The listing builds one solid part. Answer for the finished solid, in the listing's coordinates (mm). Give positions to 0.01 mm unless a question says otherwise; leave off trailing zeros. Order: outer loops, then holes, each group sorted by start corner. A loop starts at its lowest first (then second) coordinate and runs counter-clockwise, first axis right, second up. Notation, with made-up numbers: (13, 75) - (31, 75) arc R23 ccw to (31, 88) - close; hole circle Ø11 at (-11, 28). An arc over 180 degrees is marked (long way). Write each question's results on one line, items separated by ' | '. Start each with the question number.
1. Section A-A (x = 10) is taken. Give the vertices of the cut face in (y, z).
2. Find the intervals of material crossed by L1, parallel to Y at x = -63.55, z = 1.4; L2, parallel to Y at x = 40, z = 2.65; L3, parallel to Y at x = 87.1, z = 1.5, in increasing order.
3. Section B-B (z = 2.15) is taken. State how many separate pieces and enclosed holes the cut face has, and give its area (3 significant figures).
4. Determine the mould class of faces 1 (the face through (-66.498, -16.383, 1.972)), 2 (the face through (2, 27, 0)) for opening direction Y: released by +Y, released by -Y, zero draft, split by the parting line, or undercut.
5. Flat-ended cylindrical pins translate along their axes: pin 1 (4 mm diameter, centred on x = 63.55, y = 26.16, fed in from +Z); pin 2 (2 mm diameter, centred on x = 51, z = 2, fed in from -Y); pin 3 (4 mm diameter, centred on x = -40, y = -42.64, fed in from +Z); pin 4 (2 mm diameter, centred on y = -48.5, z = 1, fed in from +X). Find the tip coordinate at first contact, or state that the pin passes through.
from build123d import *

# Parameters (mm, degrees)
SKETCH1_R           = 1.5
SKETCH1_R_2         = 11
SKETCH1_R_3         = 4
SKETCH1_R_4         = 2.5
BOSS_EXTRUDE2_DEPTH = 4


with BuildPart() as part:
    # Sketch1 → Boss-Extrude2 (new body)
    with BuildSketch(Plane.XY):
        Polygon((-150.528484514, 102.663377685), (149.471515486, 102.663377685), (149.471515486, -47.336622315), (75.331349572, -47.336622315), (75.331349572, -51.336622315), (60.331349572, -51.336622315), (60.331349572, -47.336622315), (40.331349572, -47.336622315), (40.331349572, -51.336622315), (25.331349572, -51.336622315), (25.331349572, -47.336622315), (5.331349572, -47.336622315), (5.331349572, -51.336622315), (-9.668650428, -51.336622315), (-9.668650428, -47.336622315), (-29.668650428, -47.336622315), (-29.668650428, -51.336622315), (-44.668650428, -51.336622315), (-44.668650428, -47.336622315), (-63.028484514, -47.336622315), (-63.028484514, -51.336622315), (-78.028484514, -51.336622315), (-78.028484514, -47.336622315), (-150.528484514, -47.336622315), align=None)
        with Locations((-63.55, 16.163377685)):
            Circle(SKETCH1_R, mode=Mode.SUBTRACT)
        with Locations((-63.55, 26.163377685)):
            Circle(SKETCH1_R, mode=Mode.SUBTRACT)
        with Locations((-98.8, -19.086622315)):
            Circle(SKETCH1_R, mode=Mode.SUBTRACT)
        with Locations((-108.8, -19.086622315)):
            Circle(SKETCH1_R, mode=Mode.SUBTRACT)
        with Locations((63.55, 16.163377685)):
            Circle(SKETCH1_R, mode=Mode.SUBTRACT)
        with Locations((63.55, 26.163377685)):
            Circle(SKETCH1_R, mode=Mode.SUBTRACT)
        with Locations((98.8, -19.033393361)):
            Circle(SKETCH1_R, mode=Mode.SUBTRACT)
        with Locations((108.8, -19.033393361)):
            Circle(SKETCH1_R, mode=Mode.SUBTRACT)
        with Locations((64.078484514, 56.464342986)):
            Circle(SKETCH1_R_2, mode=Mode.SUBTRACT)
        with Locations((-63.55, 56.464342986)):
            Circle(SKETCH1_R_2, mode=Mode.SUBTRACT)
        with Locations((-28.3, -19.086622315)):
            Circle(SKETCH1_R, mode=Mode.SUBTRACT)
        with Locations((-18.3, -19.086622315)):
            Circle(SKETCH1_R, mode=Mode.SUBTRACT)
        with Locations((28.3, -19.086622315)):
            Circle(SKETCH1_R, mode=Mode.SUBTRACT)
        with Locations((18.3, -19.086622315)):
            Circle(SKETCH1_R, mode=Mode.SUBTRACT)
        with Locations((63.55, -19.086622315)):
            Circle(SKETCH1_R_3, mode=Mode.SUBTRACT)
        with Locations((40, 4.463377685)):
            Circle(SKETCH1_R_4, mode=Mode.SUBTRACT)
        with Locations((40, -42.636622315)):
            Circle(SKETCH1_R_4, mode=Mode.SUBTRACT)
        with Locations((87.1, 4.463377685)):
            Circle(SKETCH1_R_4, mode=Mode.SUBTRACT)
        with Locations((87.1, -42.636622315)):
            Circle(SKETCH1_R_4, mode=Mode.SUBTRACT)
        with Locations((-40, -42.636622315)):
            Circle(SKETCH1_R_4, mode=Mode.SUBTRACT)
        with Locations((-87.1, 4.463377685)):
            Circle(SKETCH1_R_4, mode=Mode.SUBTRACT)
        with Locations((-87.1, -42.636622315)):
            Circle(SKETCH1_R_4, mode=Mode.SUBTRACT)
        with Locations((-63.55, -19.086622315)):
            Circle(SKETCH1_R_3, mode=Mode.SUBTRACT)
        with Locations((-40, 4.463377685)):
            Circle(SKETCH1_R_4, mode=Mode.SUBTRACT)
    extrude(amount=BOSS_EXTRUDE2_DEPTH)


solid = part.part
Reported:
1) outline: (-47.34, 0) - (102.66, 0) - (102.66, 4) - (-47.34, 4) - close
2) L1: -51.34 to -23.09, -15.09 to 14.66, 17.66 to 24.66, 27.66 to 45.46, 67.46 to 102.66 | L2: -51.34 to -45.14, -40.14 to 1.96, 6.96 to 102.66 | L3: -47.34 to -45.14, -40.14 to 1.96, 6.96 to 102.66
3) separate pieces: 1 | enclosed holes: 24 | area: 44,200 mm²
4) face 1: undercut | face 2: zero draft
5) pin 1: z = 4 | pin 2: y = -47.34 | pin 3: through | pin 4: x = 75.33
